Autodesk Inventor part; units mm, degrees
ref_plane "YZ Plane" through (0, 0, 0) normal (1, 0, 0) x (0, 1, 0)
ref_plane "XZ Plane" through (0, 0, 0) normal (0, 1, 0) x (-1, 0, 0)
ref_plane "XY Plane" through (0, 0, 0) normal (0, 0, 1) x (1, 0, 0)
sketch "Sketch1" plane through (0, 0, 0) normal (0, 0, 1) x (1, 0, 0)
  line L0 (40.7521, 38.1) -> (40.7521, 0)
  line L1 (-60.8479, 0) -> (-60.8479, 38.1)
  line L2 (15.3521, 38.1) -> (15.3521, 63.5)
  line L3 (15.3521, 63.5) -> (-35.4479, 63.5)
  line L4 (-35.4479, 63.5) -> (-35.4479, 38.1)
  line L5 (28.0521, 0) -> (28.0521, 12.7)
  line L6 (28.0521, 12.7) -> (-48.1479, 12.7)
  line L7 (-48.1479, 12.7) -> (-48.1479, 0)
  line L8 (40.7521, 0) -> (28.0521, 0)
  line L9 (-48.1479, 0) -> (-60.8479, 0)
  line L10 (-60.8479, 38.1) -> (-35.4479, 38.1)
  line L11 (15.3521, 38.1) -> (40.7521, 38.1)
  point P0 (0, 0)
  dimension "d4" = 101.6
  dimension "d5" = 12.7
  dimension "d6" = 12.7
  dimension "d7" = 12.7
  dimension "d8" = 38.1
  dimension "d9" = 25.4
  dimension "d10" = 25.4
  dimension "d11" = 25.4
  dimension "d12" = 25.4
  dimension "d13" = 50.8
extrude "Extrusion1" add sketch "Sketch1" along normal blind 63.5
sketch "Sketch2" plane through (40.7521, 0, 0) normal (1, 0, 0) x (0, 0, -1)
  line L0 (-50.8, 19.05) -> (-12.7, 19.05)
  line L1 (-12.7, 19.05) -> (-12.7, 12.7)
  line L2 (-12.7, 12.7) -> (-50.8, 12.7)
  line L3 (-50.8, 12.7) -> (-50.8, 19.05)
  line L4 (0, 0) -> (0, 38.1)
  line L5 (0, 38.1) -> (-63.5, 38.1)
  dimension "d16" = 38.1
  dimension "d17" = 12.7
  dimension "d18" = 6.35
  dimension "d19" = 19.05
extrude "Extrusion2" add sketch "Sketch2" along normal blind 19.05
Geometry check sheet. Reference: the model listing, model coordinates, mm. A direction names the side the tool comes from. Give positions to 0.01 mm unless a question says otherwise; leave off trailing zeros. Write each loop counter-clockwise with the first axis right and the second up, starting at its lowest first coordinate (ties: lowest second). Pieces come first, ordered by that corner, then holes.
1) Go/stop test with flat-tipped pins: pin 1 Ø12 at (x, y) = (-14, 41.5) entering from -Z; pin 2 Ø7 at (x, y) = (49.5, 16) entering from +Z; pin 3 Ø1.5 at (y, z) = (47, 33.5) entering from -X; pin 4 Ø15 at (x, z) = (49.5, 39.5) entering from +Y. Record where each tip stops, or that it passes through.
Values follow:
pin 1: stops at z = 0
pin 2: stops at z = 50.8
pin 3: stops at x = -35.45
pin 4: stops at y = 19.05
2) Release check for a two-part mould opening along X. For faces 4 (the face through (28.052, 6, 31)), 5 (the face through (-10, 12.7, 31)), 6 (the face through (-35.448, 51, 31)), 7 (the face through (-11, 32, 0)) record: released by +X, released by -X, zero draft, split by the parting line, or undercut.
Values follow:
face 4: undercut
face 5: undercut
face 6: released by -X
face 7: zero draft
3) Cross-section at C-C (x = 23.5). Record the boundary of the cut face in (y, z), plus the area to 3 significant figures.
Values follow:
outline: (12.7, 0) - (38.1, 0) - (38.1, 63.5) - (12.7, 63.5) - close
area: 1,610 mm2
4) Set-up check for faces 1 (the face through (50, 16, 50.8)), 2 (the face through (50, 16, 12.7)), 3 (the face through (50, 12.7, 31)): record each of +Z, -Z, +X, -X, +Y, -Y from which the full face is reachable in a straight line by a thin tool's end or side.
Values follow:
face 1: +Z, +X, +Y, -Y
face 2: -Z, +X, +Y, -Y
face 3: +Z, -Z, +X, -Y
5) Cross-section at D-D (z = 58.5). Record the boundary of the cut face in (x, y), plus the area to 3 significant figures.
Values follow:
outline: (-60.85, 0) - (-48.15, 0) - (-48.15, 12.7) - (28.05, 12.7) - (28.05, 0) - (40.75, 0) - (40.75, 38.1) - (15.35, 38.1) - (15.35, 63.5) - (-35.45, 63.5) - (-35.45, 38.1) - (-60.85, 38.1) - close
area: 4,190 mm2
6) Cross-section at B-B (y = 48). Record the boundary of the cut face in (x, z).
Values follow:
outline: (-35.45, 0) - (15.35, 0) - (15.35, 63.5) - (-35.45, 63.5) - close
7) Cross-section at A-A (z = 21). Record the boundary of the cut face in (x, y).
Values follow:
outline: (-60.85, 0) - (-48.15, 0) - (-48.15, 12.7) - (28.05, 12.7) - (28.05, 0) - (40.75, 0) - (40.75, 12.7) - (59.8, 12.7) - (59.8, 19.05) - (40.75, 19.05) - (40.75, 38.1) - (15.35, 38.1) - (15.35, 63.5) - (-35.45, 63.5) - (-35.45, 38.1) - (-60.85, 38.1) - close
8) Thickness scan on line 1 (X direction, y = 3.5, z = 60); line 2 (X direction, y = 57, z = 40); line 3 (X direction, y = 34, z = 41). Record the ranges inside material, lowest first.
Values follow:
line 1: x = -60.85 to -48.15, 28.05 to 40.75
line 2: x = -35.45 to 15.35
line 3: x = -60.85 to 40.75
